CAD build for the part. Positions are in the model's coordinates, mm. A direction names the side the tool comes from. Give positions to 0.01 mm unless a question says otherwise; leave off trailing zeros. Write each loop counter-clockwise with the first axis right and the second up, starting at its lowest first coordinate (ties: lowest second). Pieces come first, ordered by that corner, then holes. Notation, with made-up numbers: (36.25, -36.75) -> (72.25, -36.75) arc R17 ccw to (72.25, -27.75) -> close; hole circle Ø5 at (37, 57). An arc over 180 degrees is marked (long way). Answer as a JSON object with one key per item and string values.
```python
from build123d import *

# Parameters (mm, degrees)
PAD_DEPTH       = 15
SKETCH002_W     = 44.8548
SKETCH002_H     = 24.142434
POCKET_DEPTH    = 36
SKETCH003_W     = 44.808823
SKETCH003_H     = 36
SKETCH003_R     = 1.5
PAD001_DEPTH    = 7.45
SKETCH004_R     = 5.5
SKETCH004_R_2   = 2.5
PAD002_DEPTH    = 5
SKETCH005_W     = 60
SKETCH005_H     = 20
PAD003_DEPTH    = 20
SKETCH006_W     = 40
SKETCH006_H     = 16.335257
POCKET001_DEPTH = 15


with BuildPart() as part:
    # Sketch001 → Pad (new body)
    with BuildSketch(Plane.XY):
        with BuildLine():
            ThreePointArc((-40, 18), (-58, 0), (-40, -18))
            Line((40, -18), (-40, -18))
            ThreePointArc((40, -18), (58, 0), (40, 18))
            Line((-40, 18), (40, 18))
        make_face()
    extrude(amount=PAD_DEPTH)

    # Sketch002 (on DatumPlane) → Pocket (cut)
    with BuildSketch(Plane.XZ.offset(18)):
        with Locations((0.118577, 19.728132)):
            Rectangle(SKETCH002_W, SKETCH002_H)
    extrude(amount=-POCKET_DEPTH, mode=Mode.SUBTRACT)

    # Sketch003 (on Face9 of Pocket) → Pad001 (join)
    with BuildSketch(Plane.XY.offset(7.656915)):
        with Locations((0.095588, 0)):
            Rectangle(SKETCH003_W, SKETCH003_H)
        with Locations((-18, 14)):
            Circle(SKETCH003_R, mode=Mode.SUBTRACT)
        with Locations((18, 14)):
            Circle(SKETCH003_R, mode=Mode.SUBTRACT)
        with Locations((18, -14)):
            Circle(SKETCH003_R, mode=Mode.SUBTRACT)
        with Locations((-18, -14)):
            Circle(SKETCH003_R, mode=Mode.SUBTRACT)
    extrude(amount=PAD001_DEPTH)

    # Sketch004 (on Face5 of Pad001) → Pad002 (join)
    with BuildSketch(Plane.XY.offset(15)):
        with Locations((-40, 0)):
            Circle(SKETCH004_R)
        with Locations((-40, 0)):
            Circle(SKETCH004_R_2, mode=Mode.SUBTRACT)
        with Locations((40, 0)):
            Circle(SKETCH004_R)
        with Locations((40, 0)):
            Circle(SKETCH004_R_2, mode=Mode.SUBTRACT)
    extrude(amount=PAD002_DEPTH)

    # Sketch005 (on Face4 of Pad002) → Pad003 (join)
    with BuildSketch(Plane(origin=(0, 0, 0), x_dir=(1, 0, 0), z_dir=(0, 0, -1))):
        Rectangle(SKETCH005_W, SKETCH005_H)
    extrude(amount=PAD003_DEPTH)

    # Sketch006 (on Face12 of Pad003) → Pocket001 (cut)
    with BuildSketch(Plane.XZ.offset(10)):
        with Locations((-0.04431, -10.038293)):
            Rectangle(SKETCH006_W, SKETCH006_H)
    extrude(amount=-POCKET001_DEPTH, mode=Mode.SUBTRACT)


solid = part.part
```
1) Wall check: probe 1 along Y at (x, z) = (18, 13.75); probe 2 along X at (y, z) = (1, -18); probe 3 along Z at (x, y) = (3, -5.5). Give the ranges that are in metal, low to high.
Model answer:
{"probe 1": "y = -18 to -15.5, -12.5 to 12.5, 15.5 to 18", "probe 2": "x = -30 to -20.04, 19.96 to 30", "probe 3": "z = -20 to -18.21, -1.87 to 15.11"}
2) Pin check, flat tips, straight feed: pin 1 (4 mm diameter, centred on y = -8.5, z = -9.5, fed in from +X); pin 2 (1.5 mm diameter, centred on x = 18, y = 14.5, fed in from +Z); pin 3 (7.5 mm diameter, centred on x = 6, y = -1, fed in from +Z); pin 4 (2 mm diameter, centred on y = -12.5, z = -10.5, fed in from +X). Stop position of each tip, or through.
Model answer:
{"pin 1": "stops at x = 30", "pin 2": "stops at z = 7.66", "pin 3": "stops at z = 15.11", "pin 4": "passes through"}
3) 3-axis set-ups, long thin cutter, end or side, ignore diameter. For faces 1 (the flat face through (19.956, -3, -10)), 2 (the flat face through (30, 0, -10)), 3 (the cylindrical face through (58, 0, 7)), 4 (the flat face through (-30, 0, -10)), 5 (the cylindrical face through (-45.495, 0.242, 17.465)): which of +Z, -Z, +X, -X, +Y, -Y reach the whole face in a straight line?
Model answer:
{"face 1": "-Y", "face 2": "-Z, +X, +Y, -Y", "face 3": "+Z, -Z, +X", "face 4": "-Z, -X, +Y, -Y", "face 5": "+Z"}
4) Slice it at D-D (z = -9). List the corners of the cut face in (x, y).
Model answer:
{"outline": "(-30, -10) -> (-20.04, -10) -> (-20.04, 5) -> (19.96, 5) -> (19.96, -10) -> (30, -10) -> (30, 10) -> (-30, 10) -> close"}
5) Mould opens along Z. For faces 6 (the cylindrical face through (-58, 0, 7)), 7 (the flat face through (-40, 0, 15)), 8 (the flat face through (0, -3, -18.206)) say: released by +Z, released by -Z, zero draft, split by the parting line, or undercut.
Model answer:
{"face 6": "zero draft", "face 7": "released by +Z", "face 8": "undercut"}
6) Slice it at A-A (z = 11). List the corners of the cut face in (x, y), then the cut area to 3 significant figures.
Model answer:
{"outline": "(-40, -18) -> (22.5, -18) -> (22.5, 18) -> (-40, 18) arc R18 ccw to start; (22.55, -18) -> (40, -18) arc R18 ccw to (40, 18) -> (22.55, 18) -> close; hole circle Ø3 at (-18, -14); hole circle Ø3 at (-18, 14); hole circle Ø3 at (18, -14); hole circle Ø3 at (18, 14)", "area": "3,870 mm2"}
7) Slice it at C-C (x = -18). List the corners of the cut face in (y, z), then the cut area to 3 significant figures.
Model answer:
{"outline": "(-18, 0) -> (-10, 0) -> (-10, -1.87) -> (5, -1.87) -> (5, -18.21) -> (-10, -18.21) -> (-10, -20) -> (10, -20) -> (10, 0) -> (18, 0) -> (18, 15.11) -> (15.5, 15.11) -> (15.5, 7.66) -> (12.5, 7.66) -> (12.5, 15.11) -> (-12.5, 15.11) -> (-12.5, 7.66) -> (-15.5, 7.66) -> (-15.5, 15.11) -> (-18, 15.11) -> close", "area": "654 mm2"}
